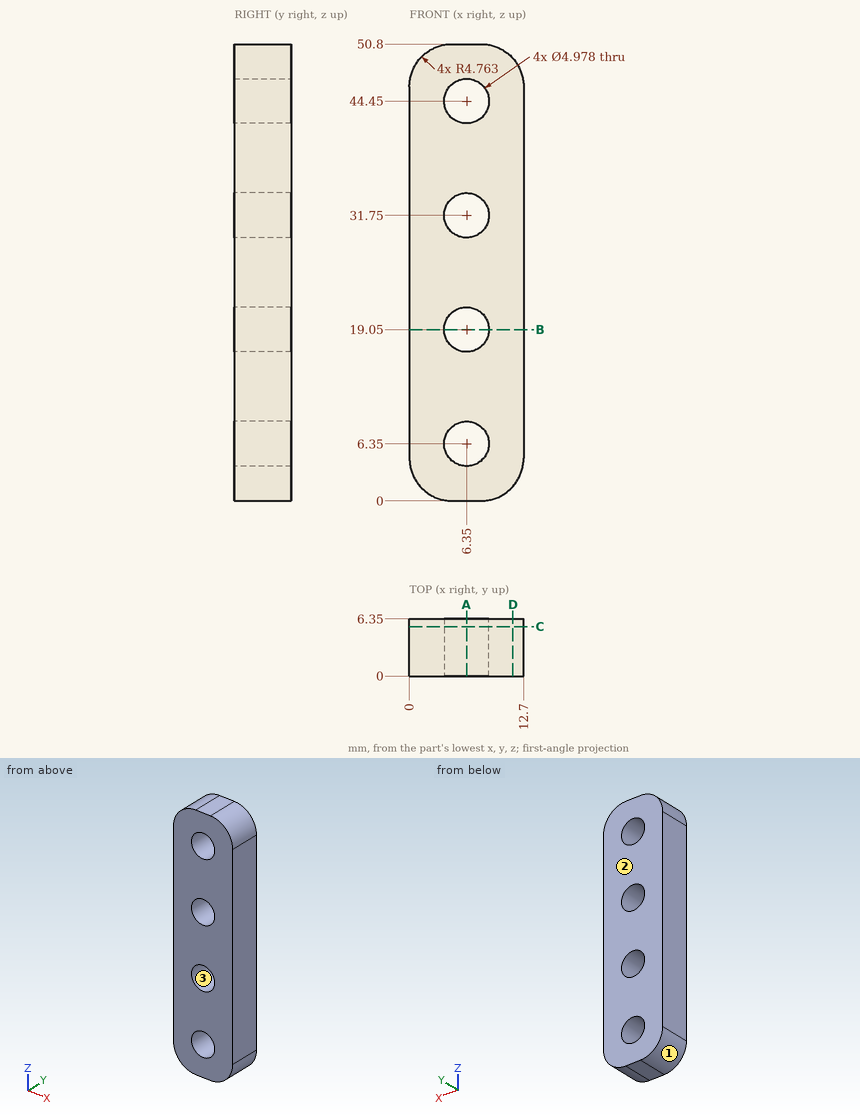
Source: three-view drawing plus pictorial views. Frame: mm from the lowest corner of the part. Round coordinates to 2 decimals unless told otherwise and drop trailing zeros. Loops run counter-clockwise (first coordinate to the right, second up) from the corner with the lowest first, then second, coordinate; pieces in that order, holes last. Notation, with made-up numbers: M 30,73 L 54,73 A18 cw 54,91 Z; hole C -11,30 d2. An arc over 180 degrees is marked long. Put each result on its own line as item: value. Start each with the question number.
(1) Draft query along Z for the marked faces 1, 2 and 3. Return one class per face: +Z half, -Z half, draft (parallel to the pull), parting line (faces both ways), or undercut.
(2) Material intervals for line 1 along X through (y, z) = (5.25, 6.35); line 2 along Z through (x, y) = (7.5, 2); line 3 along Z through (x, y) = (8.5, 3.5) (1 decimal), sorted ascending. Write a range as [from, to].
(3) Section query D-D (x = 11.5). Return loops of the section in (y, z), then the cut area to 3 significant figures.
(4) Section query C-C (y = 5.5). State how many separate pieces and enclosed holes the cut face has, then the cut area to 3 significant figures.
(5) Section query B-B (z = 19.05). Return loops of the section in (x, y).
(6) Section query A-A (x = 6.35). Return loops of the section in (y, z).
(7) Contact query for flat-ended pins moving along their axis: pin 1 Ø3 at (x, y) = (3, 4) entering from -Z; pin 2 Ø4.5 at (x, z) = (6.35, 19.05) entering from -Y. Output: stop coordinate, or through.
Findings below:
1. face 1: -Z half
1. face 2: draft
1. face 3: undercut
2. line 1: x = [0, 3.86], [8.84, 12.7]
2. line 2: z = [0, 4.14], [8.56, 16.84], [21.26, 29.54], [33.96, 42.24], [46.66, 50.8]
2. line 3: z = [0, 5.1], [7.6, 17.8], [20.3, 30.5], [33, 43.2], [45.7, 50.8]
3. outline: M 0,1.6 L 6.35,1.6 L 6.35,49.2 L 0,49.2 Z
3. area: 302 mm2
4. separate pieces: 1
4. enclosed holes: 4
4. area: 548 mm2
5. outline: M 0,0 L 3.86,0 L 3.86,6.35 L 0,6.35 Z; M 8.84,0 L 12.7,0 L 12.7,6.35 L 8.84,6.35 Z
6. outline: M 0,0 L 6.35,0 L 6.35,3.86 L 0,3.86 Z; M 0,8.84 L 6.35,8.84 L 6.35,16.56 L 0,16.56 Z; M 0,21.54 L 6.35,21.54 L 6.35,29.26 L 0,29.26 Z; M 0,34.24 L 6.35,34.24 L 6.35,41.96 L 0,41.96 Z; M 0,46.94 L 6.35,46.94 L 6.35,50.8 L 0,50.8 Z
7. pin 1: stops at z = 0.01
7. pin 2: passes through
